Study the drawing (mm; zero at the part's minimum x, y, z) and answer. Round coordinates to 2 decimals unless told otherwise and drop trailing zeros. Order: outer loops, then holes, each group sorted by start corner. A loop starts at its lowest first (then second) coordinate and runs counter-clockwise, first axis right, second up. Notation, with made-up numbers: (73, 12) -> (82, 12) arc R27 ccw to (82, 35) -> close; hole circle Ø8 at (80.25, 69). An arc over 180 degrees is marked (long way). Answer in a Markdown table with one row per item. Add a question column.
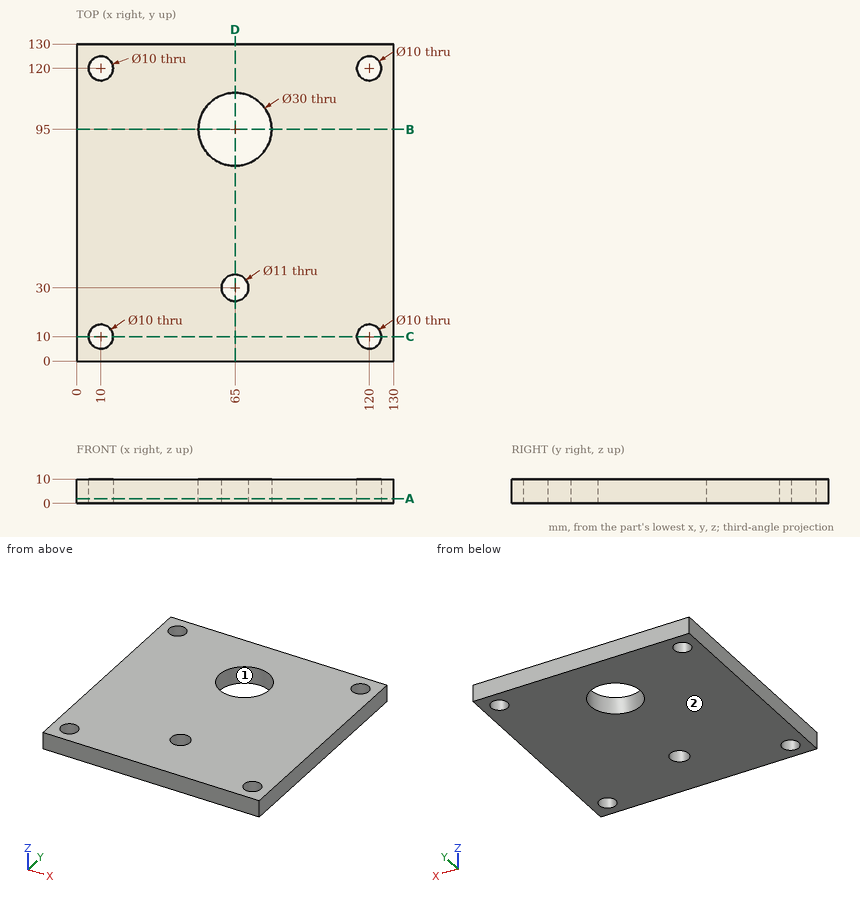
Item 1: The part is cut by section A-A, the plane z = 2. Give the vertices of the cut face in (x, y), and give its area (3 significant figures).
Item 2: The part is cut by section C-C, the plane y = 10. Give the vertices of the cut face in (x, z), and give its area (3 significant figures).
Item 3: Find the intervals of material crossed by probe 1 along Y at (x, z) = (65, 4.5); probe 2 along Y at (x, z) = (10, 4.25), in increasing order. Write a range as [from, to].
Item 4: For a pull along X with two mould halves and no side action, classify the marked faces 1 and 2 as released by +X, released by -X, zero draft, split by the parting line, or undercut.
Item 5: A flat-ended cylindrical pin translates along its axis: P1, Ø8, axis at x = 10, y = 10, coming from the +Z side. Find the tip coordinate at first contact, or state that the pin passes through.
Item 6: The part is cut by section D-D, the plane x = 65. Give the vertices of the cut face in (y, z), and give its area (3 significant figures).
Item 7: The part is cut by section B-B, the plane y = 95. Give the vertices of the cut face in (x, z).
Resolved:
| question | item | result |
|---|---|---|
| 1 | outline | (0, 0) -> (130, 0) -> (130, 130) -> (0, 130) -> close; hole circle Ø10 at (10, 10); hole circle Ø10 at (10, 120); hole circle Ø30 at (65, 95); hole circle Ø11 at (65, 30); hole circle Ø10 at (120, 10); hole circle Ø10 at (120, 120) |
| 1 | area | 15,800 mm2 |
| 2 | outline | (0, 0) -> (5, 0) -> (5, 10) -> (0, 10) -> close; (15, 0) -> (115, 0) -> (115, 10) -> (15, 10) -> close; (125, 0) -> (130, 0) -> (130, 10) -> (125, 10) -> close |
| 2 | area | 1,100 mm2 |
| 3 | probe 1 | [0, 24.5], [35.5, 80], [110, 130] |
| 3 | probe 2 | [0, 5], [15, 115], [125, 130] |
| 4 | face 1 | undercut |
| 4 | face 2 | zero draft |
| 5 | P1 | through |
| 6 | outline | (0, 0) -> (24.5, 0) -> (24.5, 10) -> (0, 10) -> close; (35.5, 0) -> (80, 0) -> (80, 10) -> (35.5, 10) -> close; (110, 0) -> (130, 0) -> (130, 10) -> (110, 10) -> close |
| 6 | area | 890 mm2 |
| 7 | outline | (0, 0) -> (50, 0) -> (50, 10) -> (0, 10) -> close; (80, 0) -> (130, 0) -> (130, 10) -> (80, 10) -> close |
